Part model, mm, in its own coordinate system. A direction names the side the tool comes from. Give positions to 0.01 mm unless a question says otherwise; leave off trailing zeros. Order: outer loops, then holes, each group sorted by start corner. A loop starts at its lowest first (then second) coordinate and runs counter-clockwise, first axis right, second up. Notation, with made-up numbers: (30.5, 2) - (44.5, 2) arc R17 ccw to (44.5, 20) - close; hole circle Ø11 at (78.25, -9.5). An arc over 180 degrees is marked (long way). One line per item, written item: value.
```python
from build123d import *

# Parameters (mm, degrees)
F2_DEPTH = 101.6
F0_R     = 36.83
F3_DEPTH = 6.35
F5_DEPTH = 6.35
F6_DEPTH = 3.175


# Not quite as in the source:
# - a feature names something its author has since deleted; it is built from what else it names


with BuildPart() as f2:
    # F1 (on face) → F2 (new body)
    with BuildSketch(Plane.YZ):
        Polygon((-28.5745194683, -8.2572300072), (-28.5730573626, -11.4344600145), (-18.8812190642, -11.43), (-6.2808282673, -11.43), (-6.2808282673, -8.2563601018), align=None)
        Polygon((0, -8.2561150224), (0, -11.43), (12.7450705782, -11.43), (28.5754804883, -11.43), (28.5754804883, -8.255), align=None)
        with BuildLine():
            Line((-14.324102157, -30.48), (-20.674102157, -30.48))
            ThreePointArc((-20.674102157, -30.48), (-10.8136603424, -35.2067273401), (0, -36.83))
            Line((0, -36.83), (0, -30.48))
            Line((0, -30.48), (-14.324102157, -30.48))
        make_face()
        with BuildLine():
            Line((0, -30.48), (0, -36.83))
            ThreePointArc((0, -36.83), (10.8136603424, -35.2067273401), (20.674102157, -30.48))
            Line((20.674102157, -30.48), (14.324102157, -30.48))
            Line((14.324102157, -30.48), (0, -30.48))
        make_face()
        Polygon((-6.2808282673, -11.43), (0, -11.43), (0, -8.2561150224), (-6.2808282673, -8.2563601018), align=None)
        Polygon((-6.2808282673, -8.2563601018), (0, -8.2561150224), (0, -5.08), (-6.2808282673, -5.08), align=None)
        with BuildLine():
            ThreePointArc((-36.4779728055, -5.08), (-35.8845812082, -8.2913045723), (-35.0090600232, -11.4374217503))
            Line((-35.0090600232, -11.4374217503), (-28.5730573626, -11.4344600145))
            Line((-28.5730573626, -11.4344600145), (-28.5745194683, -8.2572300072))
            Line((-28.5745194683, -8.2572300072), (-28.5759815739, -5.08))
            Line((-28.5759815739, -5.08), (-36.4779728055, -5.08))
        make_face()
        Polygon((-28.5759815739, -5.08), (-28.5745194683, -8.2572300072), (-6.2808282673, -8.2563601018), (-6.2808282673, -5.08), align=None)
        Polygon((0, -5.08), (0, -8.2561150224), (28.5754804883, -8.255), (28.5754804883, -5.08), align=None)
        with BuildLine():
            Line((28.5754804883, -11.43), (35.0114838303, -11.43))
            ThreePointArc((35.0114838303, -11.43), (35.8854598343, -8.2875009791), (36.4779728055, -5.08))
            Line((36.4779728055, -5.08), (28.5754804883, -5.08))
            Line((28.5754804883, -5.08), (28.5754804883, -8.255))
            Line((28.5754804883, -8.255), (28.5754804883, -11.43))
        make_face()
        with BuildLine():
            Line((14.324102157, -30.48), (20.674102157, -30.48))
            ThreePointArc((20.674102157, -30.48), (29.4269731146, -22.1472832038), (35.0114838303, -11.43))
            Line((35.0114838303, -11.43), (28.5754804883, -11.43))
            Line((28.5754804883, -11.43), (14.324102157, -30.48))
        make_face()
        with BuildLine():
            ThreePointArc((-35.0090600232, -11.4374217503), (-29.4246254725, -22.150402159), (-20.674102157, -30.48))
            Line((-20.674102157, -30.48), (-14.324102157, -30.48))
            Line((-14.324102157, -30.48), (-28.5730573626, -11.4344600145))
            Line((-28.5730573626, -11.4344600145), (-35.0090600232, -11.4374217503))
        make_face()
    extrude(amount=F2_DEPTH)

    # F0 (on Right) → F3 (join)
    with BuildSketch(Plane.YZ):
        Circle(F0_R)
    extrude(amount=-F3_DEPTH)

    # F4 (on face) → F5 (cut)
    with BuildSketch(Plane.XY.offset(-5.08)):
        Polygon((19.05, 12.7), (12.7, 12.7), (12.7, 0), (12.7, -12.7), (38.1, -12.7), (50.8, -12.7), (63.5, -12.7), (88.9, -12.7), (88.9, 0), (88.9, 12.7), (82.55, 12.7), (63.5, 12.7), (50.8, 12.7), (38.1, 12.7), align=None)
    extrude(amount=-F5_DEPTH, mode=Mode.SUBTRACT)

    # F4 (on face) → F6 (cut)
    with BuildSketch(Plane.XY.offset(-5.08)):
        Polygon((19.05, 15.875), (19.05, 12.7), (38.1, 12.7), (38.1, 15.875), (38.1, 19.05), (19.05, 19.05), align=None)
        Polygon((50.8, -12.7), (38.1, -12.7), (38.1, -15.875), (38.1, -19.05), (63.5, -19.05), (63.5, -15.875), (63.5, -12.7), align=None)
        Polygon((63.5, 15.875), (63.5, 12.7), (82.55, 12.7), (82.55, 15.875), (82.55, 19.05), (63.5, 19.05), align=None)
    extrude(amount=-F6_DEPTH, mode=Mode.SUBTRACT)


solid = f2.part
```
1) Drill centre lines: line 1 along X through (y, z) = (-18.5, -6.5); line 2 along X through (y, z) = (25.5, 6); line 3 along Z through (x, y) = (39.5, 13.5). Where is each one in solid material? Low to high. Write a range as from..to.
Outcome:
line 1: x = -6.35..38.1, 63.5..101.6
line 2: x = -6.35..0
line 3: z = -34.27..-30.48, -11.43..-5.08
2) Mould opens along Y. For faces 4 (the flat face through (38.1, 16, -7)), 5 (the flat face through (101.6, -1, -10)) say: released by +Y, released by -Y, zero draft, split by the parting line, or undercut.
Outcome:
face 4: undercut
face 5: zero draft
3) Cut at D-D, the plane y = -17.5. Give the cut face in (x, z) (3 decimals).
Outcome:
outline: (-6.35, -32.407) - (101.6, -32.407) - (101.6, -26.235) - (0, -26.235) - (0, -11.43) - (101.6, -11.43) - (101.6, -5.08) - (63.5, -5.08) - (63.5, -8.255) - (38.1, -8.255) - (38.1, -5.08) - (0, -5.08) - (0, 32.407) - (-6.35, 32.407) - close
4) Which spindle directions (+Z, -Z, +X, -X, +Y, -Y) get a long thin tool onto all of the face, cutting with end or side? Do faces 1 (the flat face through (73, 16, -8.255)), 2 (the flat face through (50, 0, -30.48)), 3 (the flat face through (0, -1, 12)). Say none if no direction does.
Outcome:
face 1: +Z
face 2: +X
face 3: +Z, +X, +Y, -Y
5) Pin check, flat tips, straight feed: pin 1 (6 mm diameter, centred on x = 10.5, y = 12.5, fed in from +Z); pin 2 (3 mm diameter, centred on x = 76.5, y = 14.5, fed in from +Z) (3 decimals); pin 3 (3.5 mm diameter, centred on x = 53.5, z = -6, fed in from +Y). Stop position of each tip, or through.
Outcome:
pin 1: stops at z = -5.08
pin 2: stops at z = -8.255
pin 3: stops at y = 36.48
6) Cut at C-C, the plane x = 50. Give the cut face in (y, z) (3 decimals).
Outcome:
outline: (-36.478, -5.08) arc R36.83 ccw to (36.478, -5.08) - (12.7, -5.08) - (12.7, -11.43) - (28.575, -11.43) - (14.324, -30.48) - (-14.324, -30.48) - (-28.573, -11.434) - (-18.881, -11.43) - (-12.7, -11.43) - (-12.7, -8.255) - (-19.05, -8.255) - (-19.05, -5.08) - close
7) Cut at A-A, the plane y = -7.5. Give the cut face in (x, z), then the cut area to 3 significant figures.
Outcome:
outline: (-6.35, -36.06) - (101.6, -36.06) - (101.6, -30.48) - (0, -30.48) - (0, -11.43) - (12.7, -11.43) - (12.7, -5.08) - (0, -5.08) - (0, 36.06) - (-6.35, 36.06) - close; (88.9, -11.43) - (101.6, -11.43) - (101.6, -5.08) - (88.9, -5.08) - close
area: 1,190 mm^2
8) Cut at B-B, the plane z = -7. Give the cut face in (x, y), then the cut area to 3 significant figures.
Outcome:
outline: (-6.35, -36.16) - (101.6, -36.16) - (101.6, 36.16) - (-6.35, 36.16) - close; hole (12.7, -12.7) - (38.1, -12.7) - (38.1, -19.05) - (63.5, -19.05) - (63.5, -12.7) - (88.9, -12.7) - (88.9, 12.7) - (82.55, 12.7) - (82.55, 19.05) - (63.5, 19.05) - (63.5, 12.7) - (38.1, 12.7) - (38.1, 19.05) - (19.05, 19.05) - (19.05, 12.7) - (12.7, 12.7) - close
area: 5,470 mm^2
